Design review of the part shown in the three views and the two pictorial views. Dimensions are in mm from the part's minimum x, y and z. Coordinates: 2 decimals unless noted, no trailing zeros. Loops run counter-clockwise (first coordinate to the right, second up) from the corner with the lowest first, then second, coordinate; pieces in that order, holes last. Notation, with made-up numbers: M 15.25,18.5 L 48.25,18.5 A5 cw 48.25,25.5 Z; hole C 38,68 d1. An arc over 180 degrees is marked long. Use one line per item in the form item = value.
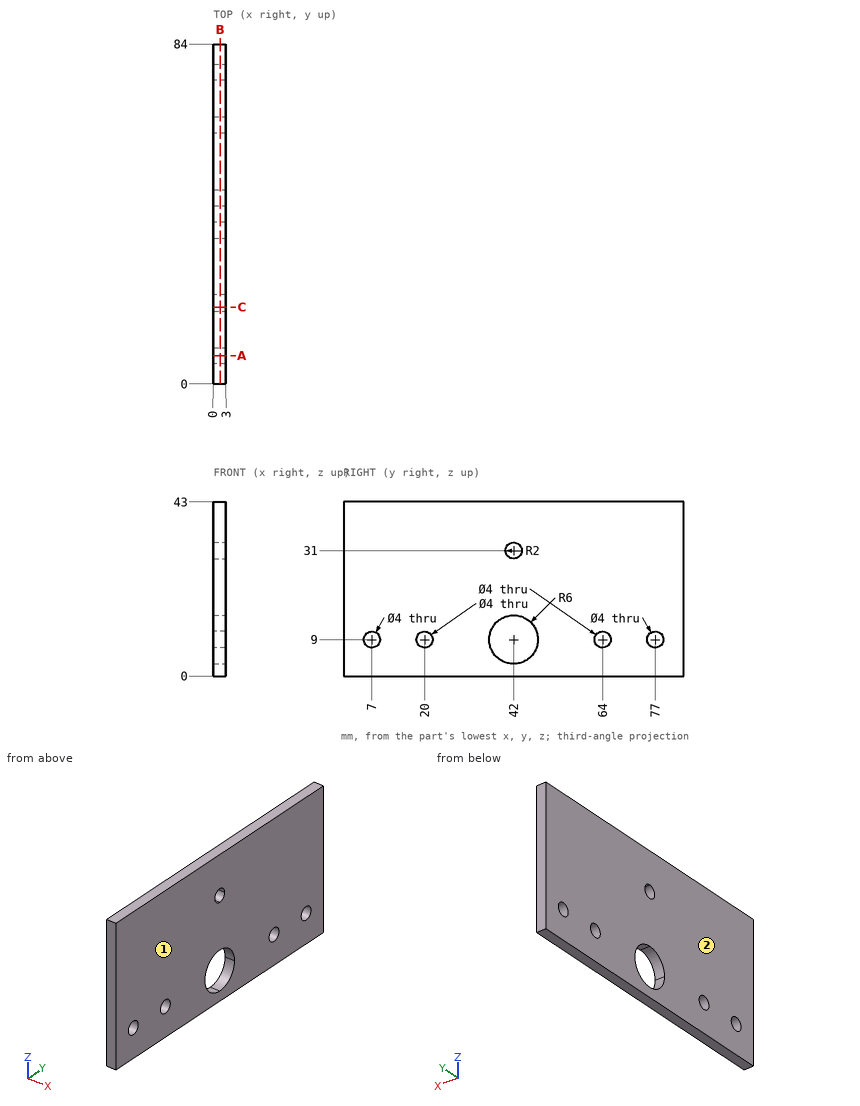
1. The part is to be moulded in two halves that separate along X. For the marked faces 1 and 2, say which applies: pulls with the +X half, pulls with the -X half, needs draft (parallel to the pull), parting line crosses it, or undercut.
Response values:
face_1 = pulls with the +X half
face_2 = pulls with the -X half
2. Insertion check: P1, Ø4.5, axis at y = 20, z = 9, coming from the +X side. The pin has a flat end and moves straight along its axis. Give the tip position at first contact, or say it passes through.
Response values:
P1 = 3
3. Add section C-C (y = 19). State the section outline as (x, z) points.
Response values:
outline = M 0,0 L 3,0 L 3,7.27 L 0,7.27 Z; M 0,10.73 L 3,10.73 L 3,43 L 0,43 Z
4. Add section B-B (x = 1.65). State the section outline as (y, z) points, then the cut area to 3 significant figures.
Response values:
outline = M 0,0 L 84,0 L 84,43 L 0,43 Z; hole C 7,9 d4; hole C 20,9 d4; hole C 42,9 d12; hole C 42,31 d4; hole C 64,9 d4; hole C 77,9 d4
area = 3,440 mm^2
5. Wall thickness on line 1 along Z through (x, y) = (1.15, 7); line 2 along Y through (x, z) = (0.25, 4); line 3 along Y through (x, z) = (1.8, 12): over which ranges is each line inside the solid? List them lowest first. Write a range as from..to.
Response values:
line_1 = 0..7, 11..43
line_2 = 0..38.68, 45.32..84
line_3 = 0..36.8, 47.2..84
6. Add section A-A (y = 7). State the section outline as (x, z) points.
Response values:
outline = M 0,0 L 3,0 L 3,7 L 0,7 Z; M 0,11 L 3,11 L 3,43 L 0,43 Z
